Model file for the job. Use its own axes, mm. A direction names the side the tool comes from. Give positions to 0.01 mm unless a question says otherwise; leave off trailing zeros. Write each loop counter-clockwise with the first axis right and the second up, starting at its lowest first coordinate (ties: lowest second). Pieces come first, ordered by that corner, then holes.
```python
from build123d import *

# Parameters (mm, degrees)
SKETCH2_R           = 9.5
SKETCH2_R_2         = 3.425
BOSS_EXTRUDE3_DEPTH = 5
BOSS_EXTRUDE5_DEPTH = 5
CIRPATTERN1_COUNT   = 10


with BuildPart() as part:
    # Sketch2 → Boss-Extrude3 (new body)
    with BuildSketch(Plane(origin=(0, 0, 0), x_dir=(0, 0, -1), z_dir=(1, 0, 0))):
        Circle(SKETCH2_R)
        Circle(SKETCH2_R_2, mode=Mode.SUBTRACT)
    extrude(amount=BOSS_EXTRUDE3_DEPTH)

    # Sketch4 → Boss-Extrude5 (add)
    with BuildSketch(Plane.ZY):
        with BuildLine():
            Line((-0.740931013, 15.366280839), (-1.685223767, 9.349332642))
            ThreePointArc((-1.685223767, 9.349332642), (0, 9.5), (1.685223767, 9.349332642))
            Line((1.685223767, 9.349332642), (0.740931013, 15.366280839))
            ThreePointArc((0.740931013, 15.366280839), (0, 16), (-0.740931013, 15.366280839))
        make_face()
    boss_extrude5 = extrude(amount=-BOSS_EXTRUDE5_DEPTH)

    # CirPattern1: Boss-Extrude5 ×10 about axis
    cirpattern1_axis = Axis((0, 0, 0), (1, 0, 0))
    for i in range(1, CIRPATTERN1_COUNT):
        add(boss_extrude5.rotate(cirpattern1_axis, i * 360 / CIRPATTERN1_COUNT))


solid = part.part
```
1. Slice it at D-D, the plane z = -4.5. Write the cut outline in (x, y), and give its area (3 significant figures).
Calculated:
outline: (0, -8.92) - (5, -8.92) - (5, 8.92) - (0, 8.92) - close
area: 89.2 mm2
2. Slice it at B-B, the plane z = 0. Write the cut outline in (x, y) (3 decimals), and give its area (3 significant figures).
Calculated:
outline: (0, -16) - (5, -16) - (5, -3.425) - (0, -3.425) - close; (0, 3.425) - (5, 3.425) - (5, 16) - (0, 16) - close
area: 126 mm2
3. Slice it at A-A, the plane y = 0. Write the cut outline in (x, z) (3 decimals), and give its area (4 significant figures).
Calculated:
outline: (0, -9.5) - (5, -9.5) - (5, -3.425) - (0, -3.425) - close; (0, 3.425) - (5, 3.425) - (5, 9.5) - (0, 9.5) - close
area: 60.75 mm2
4. Slice it at C-C, the plane y = -5. Write the cut outline in (x, z).
Calculated:
outline: (0, -15.2) - (5, -15.2) - (5, -11.55) - (0, -11.55) - close; (0, -8.08) - (5, -8.08) - (5, 8.08) - (0, 8.08) - close; (0, 11.55) - (5, 11.55) - (5, 15.2) - (0, 15.2) - close
5. Pull direction Z, two halves, no side cores. Call faces 1 (the flat face through (2.5, -9.2, -8.2)), 2 (the flat face through (2.465, 2.646, 12.09)), 3 (the cylindrical face through (2.465, 12.953, -9.392)): +Z half, -Z half, draft (parallel to the pull), parting line (faces both ways), or undercut.
Calculated:
face 1: -Z half
face 2: +Z half
face 3: undercut
6. Pin check, flat tips, straight feed: P1, Ø1, axis at x = 2, z = -8, coming from the +Y side; P2, Ø2, axis at x = 4, y = 3.5, coming from the +Z side; P3, Ø2, axis at y = 11.5, z = 11, coming from the -X side; P4, Ø1.5, axis at x = 1.5, y = 12.5, coming from the +Z side. Stop position of each tip, or through.
Calculated:
P1: stops at y = 12.93
P2: stops at z = 15.22
P3: passes through
P4: stops at z = 9.71
7. Which spindle directions (+Z, -Z, +X, -X, +Y, -Y) get a long thin tool onto all of the face, cutting with end or side? Do faces 4 (the flat face through (2.46, 10.74, 6.31)), 5 (the flat face through (2.465, 9.323, -8.265)), 6 (the cylindrical face through (2.465, -5.569, 7.696)), 7 (the flat face through (2.5, -2.7, 12.2)), 8 (the flat face through (2.46, -12.32, -1.22)). Say none if no direction does.
Calculated:
face 4: +X, -X, +Y
face 5: -Z, +X, -X
face 6: +X, -X
face 7: +Z, +X, -X
face 8: +X, -X, -Y
8. Probe probe 1 along Y at (x, z) = (1.3, 0) (3 decimals); probe 2 along Z at (x, y) = (2.25, 10); probe 3 along Y at (x, z) = (2.7, 7). List the from-to ranges inside material, lowest first.
Calculated:
probe 1: y = -16 to -3.425, 3.425 to 16
probe 2: z = -8.61 to -5.57, -1.58 to 1.58, 5.57 to 8.61
probe 3: y = -11.43 to -6.85, -6.42 to 6.42, 6.85 to 11.43
